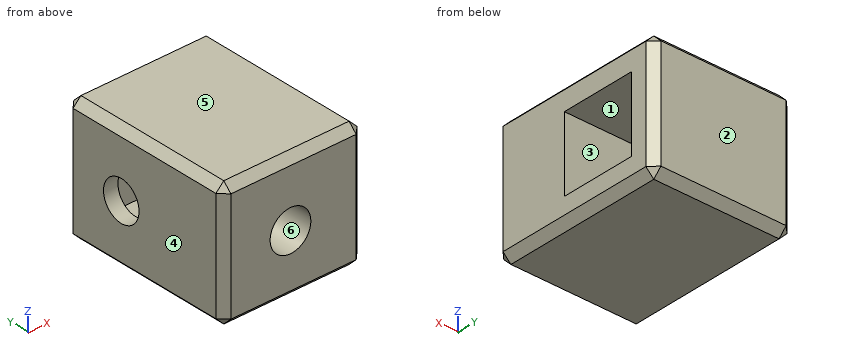
```python
from build123d import *

# Parameters (mm, degrees)
F0_W      = 17.82
F0_H      = 15.94
F1_DEPTH  = 22.2
F2_SIZE2  = 1
F2_SIZE   = 1
F3_W      = 9.48
F3_H      = 9.42
F4_DEPTH  = 16
F5_R      = 2.51
F6_DEPTH  = 25
F7_R      = 2.57
F8_DEPTH  = 6
F9_R      = 1.158766
F10_DEPTH = 1.5


with BuildPart() as f1:
    # F0 (on Front) → F1 (new body)
    with BuildSketch(Plane.XZ):
        with Locations((-8.91, 7.97)):
            Rectangle(F0_W, F0_H)
    extrude(amount=F1_DEPTH)

    # F2
    f2_edges = [f1.edges().sort_by_distance(p)[0] for p in [
        (-8.91, -22.2, 0),
        (0, -22.2, 7.97),
        (-8.91, -22.2, 15.94),
        (-17.82, -22.2, 7.97),
        (0, -11.1, 0),
        (0, -11.1, 15.94),
        (0, 0, 7.97),
        (-17.82, -11.1, 15.94),
        (-8.91, 0, 15.94),
        (-8.91, 0, 0),
        (-17.82, 0, 7.97),
        (-17.82, -11.1, 0),
    ]]
    chamfer(f2_edges, length=F2_SIZE, length2=F2_SIZE2)

    # F3 (on face) → F4 (cut)
    with BuildSketch(Plane.YZ):
        with Locations((-7.782405, 7.794221)):
            Rectangle(F3_W, F3_H)
    extrude(amount=-F4_DEPTH, mode=Mode.SUBTRACT)

    # F5 (on face) → F6 (cut)
    with BuildSketch(Plane(origin=(-17.82, 0, 0), x_dir=(0, -1, 0), z_dir=(-1, 0, 0))):
        with Locations((7.826266, 7.837604)):
            Circle(F5_R)
    extrude(amount=-F6_DEPTH, mode=Mode.SUBTRACT)

    # F7 (on face) → F8 (cut)
    with BuildSketch(Plane.XZ.offset(22.2)):
        with Locations((-9.29072, 7.7)):
            Circle(F7_R)
    extrude(amount=-F8_DEPTH, mode=Mode.SUBTRACT)

    # F9 (on face) → F10 (cut)
    with BuildSketch(Plane.XZ.offset(16.2)):
        with Locations((-9.29072, 7.7)):
            Circle(F9_R)
    extrude(amount=-F10_DEPTH, mode=Mode.SUBTRACT)


solid = f1.part
```
Build history of the part. All positions in model axes, mm. Face numbers are marked on the shaded views. A direction names the side the tool comes from. Give positions to 0.01 mm unless a question says otherwise; leave off trailing zeros. Loops run counter-clockwise (first coordinate to the right, second up) from the corner with the lowest first, then second, coordinate; pieces in that order, holes last. Notation, with made-up numbers: (78, 89) - (135, 89) arc R17 ccw to (135, 110) - close; hole circle Ø1 at (-32.5, 59.5). An arc over 180 degrees is marked (long way). Use a Markdown table: item, result.
(1) Band-saw the part on C-C (z = 4.5). Give the cut face in (x, y).
Taken from the geometry:
| item | result |
|---|---|
| outline | (-17.82, -21.2) - (-16.82, -22.2) - (-1, -22.2) - (0, -21.2) - (0, -12.52) - (-16, -12.52) - (-16, -3.04) - (0, -3.04) - (0, -1) - (-1, 0) - (-16.82, 0) - (-17.82, -1) - close |
(2) Band-saw the part on D-D (x = -11.5). Give the cut face in (y, z).
Taken from the geometry:
| item | result |
|---|---|
| outline | (-22.2, 1) - (-21.2, 0) - (-1, 0) - (0, 1) - (0, 14.94) - (-1, 15.94) - (-21.2, 15.94) - (-22.2, 14.94) - (-22.2, 9.01) - (-16.2, 9.01) - (-16.2, 6.39) - (-22.2, 6.39) - close; hole (-12.52, 3.08) - (-3.04, 3.08) - (-3.04, 12.5) - (-12.52, 12.5) - close |
(3) Wall check: line 1 along Y through (x, z) = (-12, 11.75); line 2 along Z through (x, y) = (-6.5, -11); line 3 along Y through (x, z) = (-16.75, 9.5). Give the ranges that are in metal, low to high.
Taken from the geometry:
| item | result |
|---|---|
| line 1 | -22.2 to -12.52, -3.04 to 0 |
| line 2 | 0 to 3.08, 12.5 to 15.94 |
| line 3 | -22.2 to -9.71, -5.95 to 0 |
(4) Band-saw the part on A-A (x = -2.5). Give the cut face in (y, z).
Taken from the geometry:
| item | result |
|---|---|
| outline | (-22.2, 1) - (-21.2, 0) - (-1, 0) - (0, 1) - (0, 14.94) - (-1, 15.94) - (-21.2, 15.94) - (-22.2, 14.94) - close; hole (-12.52, 3.08) - (-3.04, 3.08) - (-3.04, 12.5) - (-12.52, 12.5) - close |
(5) Band-saw the part on B-B (y = -15). Give the cut face in (x, z), and give its area (3 significant figures).
Taken from the geometry:
| item | result |
|---|---|
| outline | (-17.82, 1) - (-16.82, 0) - (-1, 0) - (0, 1) - (0, 14.94) - (-1, 15.94) - (-16.82, 15.94) - (-17.82, 14.94) - close; hole circle Ø2.32 at (-9.29, 7.7) |
| area | 278 mm2 |
(6) Which spindle directions (+Z, -Z, +X, -X, +Y, -Y) get a long thin tool onto all of the face, cutting with end or side? Do the marked faces 5 and 6. Say none if no direction does.
Taken from the geometry:
| item | result |
|---|---|
| face 5 | +Z, +X, -X, +Y, -Y |
| face 6 | -Y |
(7) Pull direction Y, two halves, no side cores. Call the marked faces 1, 2, 3 and 4: +Y half, -Y half, draft (parallel to the pull), parting line (faces both ways), or undercut.
Taken from the geometry:
| item | result |
|---|---|
| face 1 | undercut |
| face 2 | +Y half |
| face 3 | undercut |
| face 4 | draft |
(8) Drop flat-ended pins along their axis: pin 1 Ø0.7 at (x, z) = (-9.5, 7.5) entering from -Y; pin 2 Ø3 at (y, z) = (-6, 6.5) entering from +X; pin 3 Ø3 at (x, z) = (-9.29, 7.7) entering from -Y. Give the stop position or say it passes through.
Taken from the geometry:
| item | result |
|---|---|
| pin 1 | y = -14.7 |
| pin 2 | x = -16 |
| pin 3 | y = -16.2 |
